Solid Edge part; units mm, degrees
sketch "Sketch1" plane through (0, 0, 0) normal (0, 0, 1) x (1, 0, 0)
  line L0 (-308, 10) -> (308, 10)
  line L1 (308, -10) -> (-308, -10)
  arc A0 (-308, -10) -> (-308, 10) centre (-308, 0) cw
  arc A1 (308, 10) -> (308, -10) centre (308, 0) cw
  circle A2 centre (-308, 0) radius 5
  circle A3 centre (308, 0) radius 5
  circle A4 centre (0, 0) radius 5
  dimension "D1" = 308
  dimension "D2" = 308
extrude "Protrusion1" add sketch "Sketch1" against normal blind 5
Source: CAD feature listing. Evaluate the final solid. Frame: model axes, mm. Coordinates: 2 decimals unless noted, no trailing zeros. Order: outer loops, then holes, each group sorted by start corner. A loop starts at its lowest first (then second) coordinate and runs counter-clockwise, first axis right, second up. Notation, with made-up numbers: M 24.5,-31.5 L 76.5,-31.5 A21 ccw 76.5,-16.5 Z; hole C -16,4.5 d11. An arc over 180 degrees is marked long. Write each question's results on one line, items separated by ' | '. Start each with the question number.
1. Section A-A, the plane y = 0. Return the cut outline in (x, z), then the cut area to 3 significant figures.
2. Pin query (flat end, axial travel): pin 1 (8 mm diameter, centred on x = 0, y = 0, fed in from +Z); pin 2 (2 mm diameter, centred on y = 0.5, z = -2, fed in from +X). Return the tip coordinate at first contact, or that it passes through.
3. Section B-B, the plane z = -2.25. Return the cut outline in (x, y), then the cut area to 3 significant figures.
4. Material intervals for L1, parallel to X at y = -1, z = -2.35; L2, parallel to Y at x = 0, z = -1.1; L3, parallel to X at y = -2.5, z = -1.45, sorted ascending.
5. Draft query along Y for faces 1 (the face through (-303.23, 1.5, -2.46)), 2 (the face through (-318, 0, -2)), 3 (the face through (4, 5, 0)). Return one class per face: +Y half, -Y half, draft (parallel to the pull), parting line (faces both ways), or undercut.
Solution:
1) outline: M -318,-5 L -313,-5 L -313,0 L -318,0 Z; M -303,-5 L -5,-5 L -5,0 L -303,0 Z; M 5,-5 L 303,-5 L 303,0 L 5,0 Z; M 313,-5 L 318,-5 L 318,0 L 313,0 Z | area: 3,030 mm²
2) pin 1: through | pin 2: x = 318
3) outline: M -308,-10 L 308,-10 A10 ccw 308,10 L -308,10 A10 ccw Z; hole C -308,0 d10; hole C 0,0 d10; hole C 308,0 d10 | area: 12,400 mm²
4) L1: -317.95 to -312.9, -303.1 to -4.9, 4.9 to 303.1, 312.9 to 317.95 | L2: -10 to -5, 5 to 10 | L3: -317.68 to -312.33, -303.67 to -4.33, 4.33 to 303.67, 312.33 to 317.68
5) face 1: undercut | face 2: parting line | face 3: draft
